For this review, take the finished solid that the model builds, in its own axes (mm). Face numbers are marked on the shaded views. A direction names the side the tool comes from. Round coordinates to 2 decimals unless told otherwise and drop trailing zeros. Write each loop counter-clockwise with the first axis right and the second up, starting at its lowest first coordinate (ties: lowest second). Pieces come first, ordered by that corner, then holes. Notation, with made-up numbers: (50, 9) - (105, 9) arc R25 ccw to (105, 40) - close; hole circle Ø3 at (54, 16). An arc over 180 degrees is marked (long way). One line per item, written item: value. Start each with the question number.
Q1. For probe 1 along X at (y, z) = (5, -0.75); probe 2 along Y at (x, z) = (4.5, 6.25); probe 3 along X at (y, z) = (3, 1.25), list the stretches that pass through material, from the lowest coordinate up.
Q2. Clearance check with flat-ended pins moving along their axes: pin 1 Ø4 at (x, y) = (37.5, 4) entering from +Z; pin 2 Ø5 at (x, y) = (38, 3) entering from +Z; pin 3 Ø1 at (y, z) = (-6, -2.5) entering from -X. State where each tip first meets the part, or that it passes through.
Q3. Tool access review of the marked faces 1, 2 and 3: name each direction out of +Z, -Z, +X, -X, +Y, -Y from which nothing blocks a thin tool from reaching the whole face with its end or side.
Q4. Add section A-A on x = 29.5. Write out the cut boundary in (y, z).
Q5. Add section B-B on y = -5.25. Write out the cut boundary in (x, z).
```python
from build123d import *

# Parameters (mm, degrees)
SKETCH1_R           = 7.25
BOSS_EXTRUDE1_DEPTH = 49.4
SKETCH2_R           = 2.75
BOSS_EXTRUDE2_DEPTH = 1
SKETCH3_R           = 3.5
BOSS_EXTRUDE3_DEPTH = 0.1
FILLET1_R           = 0.2


with BuildPart() as part:
    # Sketch1 → Boss-Extrude1 (new body)
    with BuildSketch(Plane(origin=(0, 0, 0), x_dir=(0, 0, -1), z_dir=(1, 0, 0))):
        Circle(SKETCH1_R)
    extrude(amount=BOSS_EXTRUDE1_DEPTH)

    # Sketch2 → Boss-Extrude2 (add)
    with BuildSketch(Plane(origin=(49.4, 0, 0), x_dir=(0, 0, -1), z_dir=(1, 0, 0))):
        Circle(SKETCH2_R)
    extrude(amount=BOSS_EXTRUDE2_DEPTH)

    # Sketch3 → Boss-Extrude3 (add)
    with BuildSketch(Plane.ZY):
        with Locations(Location((0, 0, 0), (0, 0, 180))):
            Circle(SKETCH3_R)
    extrude(amount=BOSS_EXTRUDE3_DEPTH)

    # Fillet1
    # the kernel refuses this fillet: 0.2 mm, written as the material it adds along each edge
    with BuildSketch(Plane(origin=(0, 0, 0), x_dir=(0, 0, -1), z_dir=(0, 1, 0))) as fillet1_piece_1:
        with BuildLine():
            CenterArc((3.673205081, 0.2), FILLET1_R, 210, 60)
            Line((3.5, 0.1), (3.496535898, 0.098))
            ThreePointArc((3.496535898, 0.098), (3.496, 0.05), (3.496, 0))
            Line((3.496, 0), (3.5, -0.004))
            Line((3.5, -0.004), (3.673205081, -0.004))
            Line((3.673205081, -0.004), (3.673205081, 0))
        make_face()
    revolve(axis=Axis((0, 0, 0), (-1, 0, 0)))


solid = part.part
```
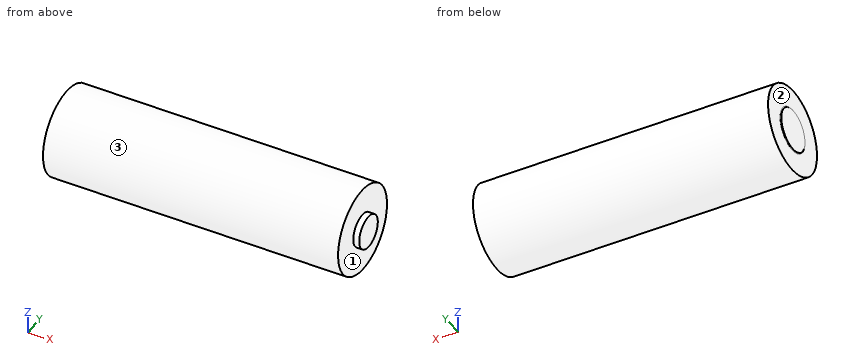
Result set:
1. probe 1: x = 0 to 49.4
1. probe 2: y = -3.67 to 3.67
1. probe 3: x = -0.1 to 49.4
2. pin 1: stops at z = 6.97
2. pin 2: stops at z = 7.23
2. pin 3: stops at x = 0
3. face 1: +X
3. face 2: -X
3. face 3: +X, -X
4. outline: circle Ø14.5 at (0, 0)
5. outline: (0, -5) - (49.4, -5) - (49.4, 5) - (0, 5) - close
